Read the model definition and answer for the solid it produces. Units are mm, in the model's axes. Coordinates: 2 decimals unless noted, no trailing zeros. Order: outer loops, then holes, each group sorted by start corner. A loop starts at its lowest first (then second) coordinate and runs counter-clockwise, first axis right, second up. Notation, with made-up numbers: (57, 25.5) -> (90, 25.5) arc R21 ccw to (90, 53.5) -> close; hole circle Ø9 at (13, 17.5). An arc over 180 degrees is marked (long way). Answer as a JSON object with one key per item and string values. Group by question number.
1) Section B-B on y = 2.15 is taken. Count the separate pieces of the cut face and the enclosed holes in it, and give its area (3 significant figures).
2) Section A-A on x = -41.5 is taken. Determine the outline of the cut face in (y, z), and give its area (3 significant figures).
3) Given pin 1 (0.9 mm diameter, centred on x = 32, y = 1, fed in from -Z); pin 2 (1.5 mm diameter, centred on x = -30, y = 1, fed in from +Z), each flat-ended and moving along its own axis, determine where each tip first touches the part or whether it passes through.
4) Consider L1, parallel to X at y = 0.8, z = -36.5; L2, parallel to Z at x = -43, y = 2.35; L3, parallel to X at y = 0.95, z = 32. Determine where each line is inside the solid, lowest interval first.
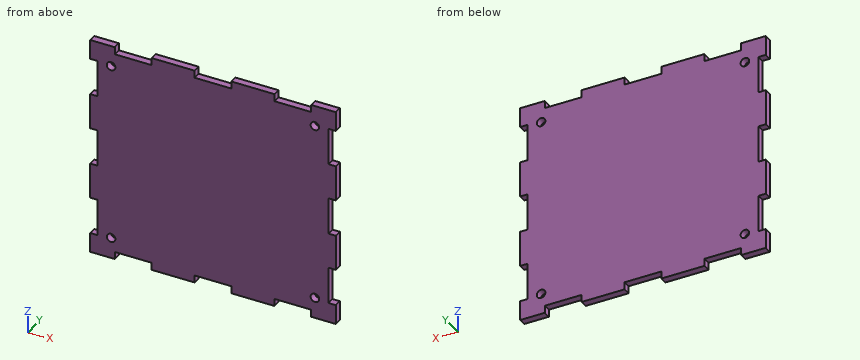
from build123d import *

# Parameters (mm, degrees)
SKETCH_1_R      = 1.75
EXTRUDE_1_DEPTH = 3


with BuildPart() as part:
    # 草图1 → 凸台-拉伸1 (new body)
    with BuildSketch(Plane(origin=(0, 0, 0), x_dir=(1, 0, 0), z_dir=(0, 1, 0))):
        Polygon((-50, -45), (-40, -45), (-40, -42), (-25, -42), (-25, -45), (-7.5, -45), (-7.5, -42), (7.5, -42), (7.5, -45), (25, -45), (25, -42), (40, -42), (40, -45), (50, -45), (50, -37), (47, -37), (47, -22), (50, -22), (50, -7.5), (47, -7.5), (47, 7.5), (50, 7.5), (50, 22), (47, 22), (47, 37), (50, 37), (50, 45), (40, 45), (40, 42), (25, 42), (25, 45), (7.5, 45), (7.5, 42), (-7.5, 42), (-7.5, 45), (-25, 45), (-25, 42), (-40, 42), (-40, 45), (-50, 45), (-50, 37), (-47, 37), (-47, 22), (-50, 22), (-50, 7.5), (-47, 7.5), (-47, -7.5), (-50, -7.5), (-50, -22), (-47, -22), (-47, -37), (-50, -37), align=None)
        with Locations(Location((-41.5, 36.5, 0), (0, 0, 270))):
            Circle(SKETCH_1_R, mode=Mode.SUBTRACT)
        with Locations(Location((41.5, 36.5, 0), (0, 0, 270))):
            Circle(SKETCH_1_R, mode=Mode.SUBTRACT)
        with Locations(Location((41.5, -36.5, 0), (0, 0, 270))):
            Circle(SKETCH_1_R, mode=Mode.SUBTRACT)
        with Locations(Location((-41.5, -36.5, 0), (0, 0, 270))):
            Circle(SKETCH_1_R, mode=Mode.SUBTRACT)
    extrude(amount=EXTRUDE_1_DEPTH)


solid = part.part
Worked answers:
{
 "1": {"separate pieces": "1", "enclosed holes": "4", "area": "8,420 mm²"},
 "2": {"outline": "(0, -45) -> (3, -45) -> (3, -38.25) -> (0, -38.25) -> close; (0, -34.75) -> (3, -34.75) -> (3, 34.75) -> (0, 34.75) -> close; (0, 38.25) -> (3, 38.25) -> (3, 45) -> (0, 45) -> close", "area": "249 mm²"},
 "3": {"pin 1": "stops at z = -42", "pin 2": "stops at z = 42"},
 "4": {"L1": "x = -47 to -43.25, -39.75 to 39.75, 43.25 to 47", "L2": "z = -45 to -37.4, -35.6 to 35.6, 37.4 to 45", "L3": "x = -47 to 47"}
}
